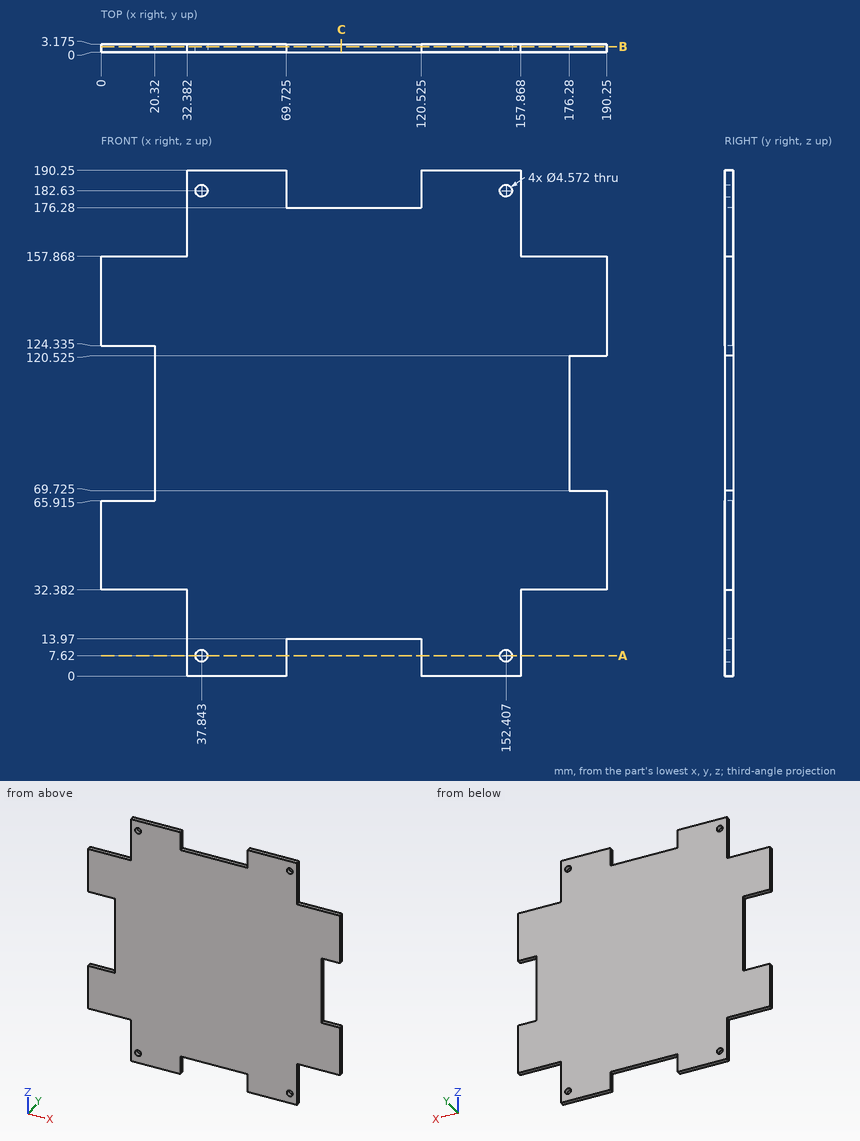
Study the drawing (mm; zero at the part's minimum x, y, z) and answer. Coordinates: 2 decimals unless noted, no trailing zeros. Write each loop counter-clockwise with the first axis right and the second up, starting at its lowest first coordinate (ties: lowest second). Pieces come first, ordered by that corner, then holes. Notation, with made-up numbers: (-16.5, 63) - (19.5, 63) arc R28 cw to (19.5, 86) - close; hole circle Ø5 at (23, 40). An arc over 180 degrees is marked (long way). Answer as a JSON object with one key per item and string values. Group by question number.
1. A cutting plane is placed at B-B (y = 2.2). Give the number of separate pieces and of enclosed holes in the cut face, plus the area to 3 significant figures.
2. Each of these flat-tipped pins is pushed along its axis until it touches: P1, Ø1.6, axis at y = 2, z = 16.5, coming from the -X side; P2, Ø1, axis at y = 2, z = 89.5, coming from the +X side; P3, Ø1, axis at x = 88, y = 2.5, coming from the -Z side. Where does it stop, or does it pass through?
3. A cutting plane is placed at C-C (x = 90.5). Determine the outline of the cut face in (y, z) (3 decimals), plus the area to 3 significant figures.
4. A cutting plane is placed at A-A (z = 7.62). Determine the outline of the cut face in (x, y) (3 decimals), plus the area to 3 significant figures.
5. Consider L1, parallel to X at y = 1.75, z = 182.63 (3 decimals); L2, parallel to Z at x = 11, y = 0.25 (3 decimals); L3, parallel to X at y = 1.6, z = 9.5 (3 decimals). Determine where each line is inside the solid, lowest interval first. Write a range as [from, to].
Worked out:
{
 "1": {"separate pieces": "1", "enclosed holes": "4", "area": "28,600 mm²"},
 "2": {"P1": "stops at x = 32.38", "P2": "stops at x = 176.28", "P3": "stops at z = 13.97"},
 "3": {"outline": "(0, 13.97) - (3.175, 13.97) - (3.175, 176.28) - (0, 176.28) - close", "area": "515 mm²"},
 "4": {"outline": "(32.382, 0) - (35.557, 0) - (35.557, 3.175) - (32.382, 3.175) - close; (40.129, 0) - (69.725, 0) - (69.725, 3.175) - (40.129, 3.175) - close; (120.525, 0) - (150.121, 0) - (150.121, 3.175) - (120.525, 3.175) - close; (154.693, 0) - (157.868, 0) - (157.868, 3.175) - (154.693, 3.175) - close", "area": "208 mm²"},
 "5": {"L1": "x = [32.382, 35.557], [40.129, 69.725], [120.525, 150.121], [154.693, 157.868]", "L2": "z = [32.382, 65.915], [124.335, 157.868]", "L3": "x = [32.382, 36.542], [39.144, 69.725], [120.525, 151.106], [153.708, 157.868]"}
}
